from build123d import *

# Parameters (mm, degrees)
F3_R      = 4.5
F4_DEPTH  = 42.5
F8_DEPTH  = 42.5
F6_R      = 4.5
F6_R_2    = 4
F9_DEPTH  = 22.5
F7_R      = 4.5
F7_R_2    = 4
F10_DEPTH = 11
F11_R     = 2.5
F11_R_2   = 0.75
F12_DEPTH = 4.501


# Not quite as in the source:
# - ends of sketch curves that miss each other by under 0.0002 mm in the source are joined


with BuildPart() as f4:
    # F3 (on Front) → F4 (new body)
    with BuildSketch(Plane.XZ):
        Circle(F3_R)
    extrude(amount=F4_DEPTH)

    # F5 (on face) → F8 (cut, through all)
    with BuildSketch(Plane.XZ.offset(42.5)):
        with BuildLine():
            Line((-1.25, -3.8), (0, -3.8))
            Line((0, -3.8), (1.25, -3.8))
            Line((1.25, -3.8), (1.25, -3.7))
            ThreePointArc((1.25, -3.7), (1.3085786438, -3.5585786438), (1.45, -3.5))
            Line((1.45, -3.5), (2, -3.5))
            Line((2, -3.5), (2, -3.05))
            ThreePointArc((2, -3.05), (2.0585786438, -2.9085786438), (2.2, -2.85))
            Line((2.2, -2.85), (3.15, -2.85))
            Line((3.15, -2.85), (3.15, -2.15))
            Line((3.15, -2.15), (2.2, -2.15))
            ThreePointArc((2.2, -2.15), (2.0585786438, -2.0914213562), (2, -1.95))
            Line((2, -1.95), (2, -1.887459))
            ThreePointArc((2, -1.887459), (2.1033535752, -1.771554046), (2.2, -1.65))
            Line((2.2, -1.65), (3.75, -1.65))
            Line((3.75, -1.65), (3.75, 0))
            Line((3.75, 0), (3.75, 1.65))
            Line((3.75, 1.65), (2.2, 1.65))
            ThreePointArc((2.2, 1.65), (2.1033535752, 1.771554046), (1.9999998047, 1.8874588157))
            Line((1.9999998047, 1.8874588157), (2, 1.95))
            ThreePointArc((2, 1.95), (2.0585786438, 2.0914213562), (2.2, 2.15))
            Line((2.2, 2.15), (3.15, 2.15))
            Line((3.15, 2.15), (3.15, 2.85))
            Line((3.15, 2.85), (2.2, 2.85))
            ThreePointArc((2.2, 2.85), (2.0585786438, 2.9085786438), (2, 3.05))
            Line((2, 3.05), (2, 3.5))
            Line((2, 3.5), (1.45, 3.5))
            ThreePointArc((1.45, 3.5), (1.3085786438, 3.5585786438), (1.25, 3.7))
            Line((1.25, 3.7), (1.25, 3.8))
            Line((1.25, 3.8), (0, 3.8))
            Line((0, 3.8), (-1.25, 3.8))
            Line((-1.25, 3.8), (-1.25, 3.7))
            ThreePointArc((-1.25, 3.7), (-1.3085786438, 3.5585786438), (-1.45, 3.5))
            Line((-1.45, 3.5), (-2, 3.5))
            Line((-2, 3.5), (-2, 3.05))
            ThreePointArc((-2, 3.05), (-2.0585786438, 2.9085786438), (-2.2, 2.85))
            Line((-2.2, 2.85), (-3.15, 2.85))
            Line((-3.15, 2.85), (-3.15, 2.15))
            Line((-3.15, 2.15), (-2.2, 2.15))
            ThreePointArc((-2.2, 2.15), (-2.0585786438, 2.0914213562), (-2, 1.95))
            Line((-2, 1.95), (-2, 1.887459))
            ThreePointArc((-2, 1.887459), (-2.1033535752, 1.771554046), (-2.2, 1.65))
            Line((-2.2, 1.65), (-3.75, 1.65))
            Line((-3.75, 1.65), (-3.75, 0))
            Line((-3.75, 0), (-3.75, -1.65))
            Line((-3.75, -1.65), (-2.2, -1.65))
            ThreePointArc((-2.2, -1.65), (-2.1033535752, -1.771554046), (-1.9999998047, -1.8874588157))
            Line((-1.9999998047, -1.8874588157), (-2, -1.95))
            ThreePointArc((-2, -1.95), (-2.0585786438, -2.0914213562), (-2.2, -2.15))
            Line((-2.2, -2.15), (-3.15, -2.15))
            Line((-3.15, -2.15), (-3.15, -2.85))
            Line((-3.15, -2.85), (-2.2, -2.85))
            ThreePointArc((-2.2, -2.85), (-2.0585786438, -2.9085786438), (-2, -3.05))
            Line((-2, -3.05), (-2, -3.5))
            Line((-2, -3.5), (-1.45, -3.5))
            ThreePointArc((-1.45, -3.5), (-1.3085786438, -3.5585786438), (-1.25, -3.7))
            Line((-1.25, -3.7), (-1.25, -3.8))
        make_face()
    extrude(amount=-F8_DEPTH, mode=Mode.SUBTRACT)

    # F6 (on face) → F9 (join)
    with BuildSketch(Plane.XZ.offset(42.5)):
        Circle(F6_R)
        Circle(F6_R_2, mode=Mode.SUBTRACT)
    extrude(amount=F9_DEPTH)

    # F7 (on face) → F10 (join)
    with BuildSketch(Plane(origin=(0, 0, 0), x_dir=(-1, 0, 0), z_dir=(0, 1, 0))):
        Circle(F7_R)
        Circle(F7_R_2, mode=Mode.SUBTRACT)
    extrude(amount=F10_DEPTH)

    # F11 (on Right) → F12 (cut, through all)
    with BuildSketch(Plane.YZ):
        with Locations((-59, 0)):
            Circle(F11_R)
        with Locations((-63.25, 0)):
            Circle(F11_R_2)
    extrude(amount=-F12_DEPTH, mode=Mode.SUBTRACT)


solid = f4.part
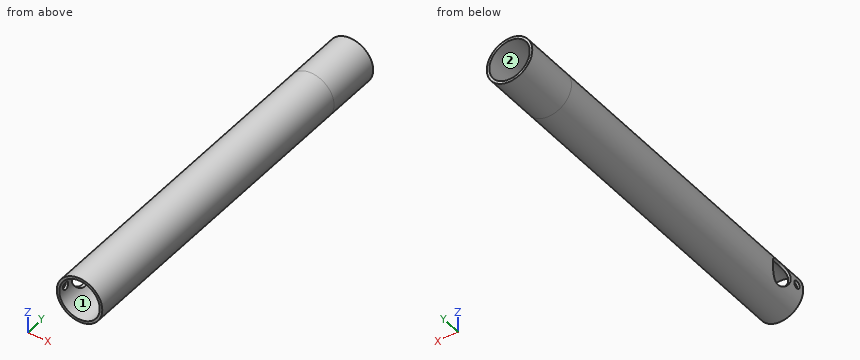
Work out the finished part from the listing and answer in its coordinate system (mm). Face numbers are marked on the shaded views. Coordinates: 2 decimals unless noted, no trailing zeros. Loops run counter-clockwise (first coordinate to the right, second up) from the corner with the lowest first, then second, coordinate; pieces in that order, holes last. Notation, with made-up numbers: M -33,9 L -27,9 A26 cw -27,38 Z; hole C -24.75,74.25 d11. An arc over 180 degrees is marked long. Answer in a Markdown table with one row per item. Add a question column.
1. Consider L1, parallel to Z at x = 0, y = 7.25; L2, parallel to Z at x = 0, y = -14.5. Determine where each line is inside the solid, lowest interval first.
2. Find section C-C, the plane y = -49. Write down the section's boundary in (x, z), then the cut area to 3 significant figures.
3. Find section D-D, the plane y = -59. Write down the section's boundary in (x, z), then the cut area to 3 significant figures.
4. The mould has two halves that part along Z. Classify the marked faces 1 and 2: pulls with the +Z half, pulls with the -Z half, needs draft (parallel to the pull), parting line crosses it, or undercut.
5. Flat-ended cylindrical pins translate along their axes: P1, Ø0.8, axis at x = -3, y = -11.5, coming from the -Z side; P2, Ø2, axis at y = -46, z = 0.5, coming from the -X side; P3, Ø0.9, axis at x = -2.5, z = -2, coming from the +Y side; P4, Ø1.4, axis at y = -63.25, z = 0, coming from the -X side. Find the tip coordinate at first contact, or state that the pin passes through.
6. Find section B-B, the plane x = 0. Write down the section's boundary in (y, z), then the cut area to 3 significant figures.
7. Find section A-A, the plane z = 0. Write down the section's boundary in (x, y).
Reported:
| question | item | result |
|---|---|---|
| 1 | L1 | z = -4.5 to -4, 4 to 4.5 |
| 1 | L2 | z = -4.5 to -3.8, 3.8 to 4.5 |
| 2 | outline | C 0,0 d9; hole C 0,0 d8 |
| 2 | area | 13.4 mm^2 |
| 3 | outline | M -3.74,-2.5 A4.5 ccw long -3.74,2.5 L -3.12,2.5 A4 cw long -3.12,-2.5 Z |
| 3 | area | 10.7 mm^2 |
| 4 | face 1 | undercut |
| 4 | face 2 | undercut |
| 5 | P1 | stops at z = -3.67 |
| 5 | P2 | stops at x = -4.5 |
| 5 | P3 | stops at y = 0 |
| 5 | P4 | stops at x = 3.94 |
| 6 | outline | M -65,-4.5 L 11,-4.5 L 11,-4 L 0,-4 L 0,-3.8 L -42.5,-3.8 L -42.5,-4 L -65,-4 Z; M -65,4 L -42.5,4 L -42.5,3.8 L 0,3.8 L 0,4 L 11,4 L 11,4.5 L -65,4.5 Z |
| 6 | area | 93.0 mm^2 |
| 7 | outline | M -4.5,-65 L -4,-65 L -4,-64 L -4.5,-64 Z; M -4.5,-62.5 L -4,-62.5 L -4,-61.5 L -4.5,-61.5 Z; M -4.5,-56.5 L -4,-56.5 L -4,-42.5 L -3.75,-42.5 L -3.75,0 L -4,0 L -4,11 L -4.5,11 Z; M 3.75,-42.5 L 4,-42.5 L 4,-65 L 4.5,-65 L 4.5,11 L 4,11 L 4,0 L 3.75,0 Z |
